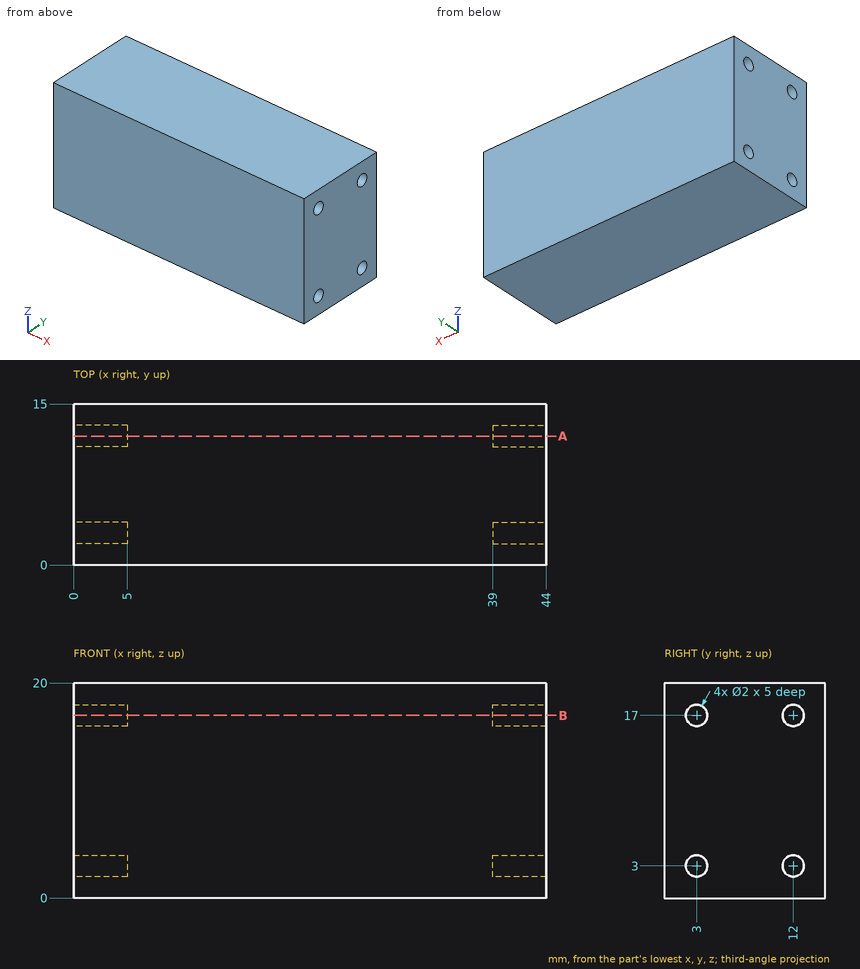
Study the drawing (mm; zero at the part's minimum x, y, z) and answer. Give positions to 0.01 mm unless a question says otherwise; leave off trailing zeros. Loops run counter-clockwise (first coordinate to the right, second up) from the corner with the lowest first, then second, coordinate; pieces in that order, holes last. Notation, with made-up numbers: (5.25, 21) - (59.25, 21) arc R24 cw to (59.25, 45) - close; hole circle Ø6 at (32.25, -3.75). An arc over 180 degrees is marked (long way). Answer in a Markdown table with one row per item. Add a question column.
Q1. Each of these flat-tipped pins is pushed along its axis until it touches: P1, Ø1.8, axis at y = 12, z = 17, coming from the -X side; P2, Ø1, axis at y = 2.5, z = 17.5, coming from the +X side; P3, Ø1.2, axis at y = 3, z = 3, coming from the +X side. Where does it stop, or does it pass through?
Q2. Consider line 1 along Y through (x, z) = (3.3, 3). Determine where the line is inside the solid, lowest interval first.
Q3. The part is cut by section B-B (z = 17). Determine the outline of the cut face in (x, y).
Q4. The part is cut by section A-A (y = 12). Determine the outline of the cut face in (x, z).
Solution:
| question | item | result |
|---|---|---|
| 1 | P1 | stops at x = 5 |
| 1 | P2 | stops at x = 44 |
| 1 | P3 | stops at x = 39 |
| 2 | line 1 | y = 0 to 2, 4 to 11, 13 to 15 |
| 3 | outline | (0, 0) - (44, 0) - (44, 2) - (39, 2) - (39, 4) - (44, 4) - (44, 11) - (39, 11) - (39, 13) - (44, 13) - (44, 15) - (0, 15) - (0, 13) - (5, 13) - (5, 11) - (0, 11) - (0, 4) - (5, 4) - (5, 2) - (0, 2) - close |
| 4 | outline | (0, 0) - (44, 0) - (44, 2) - (39, 2) - (39, 4) - (44, 4) - (44, 16) - (39, 16) - (39, 18) - (44, 18) - (44, 20) - (0, 20) - (0, 18) - (5, 18) - (5, 16) - (0, 16) - (0, 4) - (5, 4) - (5, 2) - (0, 2) - close |
